Autodesk Inventor part; units mm, degrees
ref_plane "YZ Plane" through (0, 0, 0) normal (1, 0, 0) x (0, 1, 0)
ref_plane "XZ Plane" through (0, 0, 0) normal (0, 1, 0) x (-1, 0, 0)
ref_plane "XY Plane" through (0, 0, 0) normal (0, 0, 1) x (1, 0, 0)
sketch "スケッチ1" plane through (0, 0, 0) normal (0, 0, 1) x (1, 0, 0)
  point P0 (0, 0)
sketch "スケッチ2" plane through (0, 0, 0) normal (0, 0, 1) x (1, 0, 0)
  line L0 (72.5, -37.5) -> (-72.5, -37.5)
  line L1 (-72.5, -37.5) -> (-72.5, 37.5)
  line L2 (-72.5, 37.5) -> (72.5, 37.5)
  line L3 (72.5, 37.5) -> (72.5, -37.5)
  line L4 (72.5, -37.5) -> (-72.5, 37.5) construction
  line L5 (-72.5, -37.5) -> (72.5, 37.5) construction
  circle A0 centre (-48, -17) radius 6.05
  circle A1 centre (-48, -17) radius 9
  circle A2 centre (-57, -17) radius 1.6
  circle A3 centre (-48, -26) radius 1.6
  circle A4 centre (-39, -17) radius 1.6
  circle A5 centre (-48, -8) radius 1.6
  line L6 (67.5, 32.5) -> (-67.5, 32.5)
  line L7 (-67.5, 32.5) -> (-67.5, -32.5)
  line L8 (-67.5, -32.5) -> (67.5, -32.5)
  line L9 (67.5, -32.5) -> (67.5, 32.5)
  line L10 (-67.5, 32.5) -> (-67.5, 12.5) construction
  line L11 (-69.1, 32.5) -> (-69.1, 12.5)
  line L12 (-65.9, 12.5) -> (-65.9, 32.5)
  arc A6 (-65.9, 32.5) -> (-69.1, 32.5) centre (-67.5, 32.5) ccw
  arc A7 (-69.1, 12.5) -> (-65.9, 12.5) centre (-67.5, 12.5) ccw
  line L13 (-67.5, 32.5) -> (-47.5, 32.5) construction
  line L14 (-67.5, -32.5) -> (-67.5, -12.5) construction
  line L15 (-65.9, -32.5) -> (-65.9, -12.5)
  line L16 (-69.1, -12.5) -> (-69.1, -32.5)
  arc A8 (-69.1, -32.5) -> (-65.9, -32.5) centre (-67.5, -32.5) ccw
  arc A9 (-65.9, -12.5) -> (-69.1, -12.5) centre (-67.5, -12.5) ccw
  line L17 (-67.5, -32.5) -> (-47.5, -32.5) construction
  line L18 (67.5, 32.5) -> (105, 32.5) construction
  line L19 (-72.5, -17) -> (72.5, -17)
  circle A10 centre (0, -17) radius 9
  circle A11 centre (0, -17) radius 39
  line L20 (-65, 37.5) -> (65, 37.5)
  line L21 (65, 37.5) -> (65, 32.5)
  line L22 (65, 32.5) -> (-65, 32.5)
  line L23 (-65, 32.5) -> (-65, 37.5)
  line L24 (-65, 32.5) -> (0, 0)
  line L25 (0, 0) -> (65, 32.5)
  line L26 (-72.5, 0) -> (72.5, 0)
  line L27 (72.5, 0) -> (72.5, -47.5)
  line L28 (72.5, -47.5) -> (-72.5, -47.5)
  line L29 (-72.5, -47.5) -> (-72.5, 0)
  circle A12 centre (-67.5, 32.5) radius 1.6
  circle A13 centre (-67.5, -12.5) radius 1.6
  line L30 (0, 37.5) -> (0, -47.5)
  line L31 (67.5, 32.5) -> (67.5, 12.5) construction
  line L32 (69.1, 32.5) -> (69.1, 12.5)
  line L33 (65.9, 12.5) -> (65.9, 32.5)
  arc A14 (69.1, 32.5) -> (65.9, 32.5) centre (67.5, 32.5) ccw
  arc A15 (65.9, 12.5) -> (69.1, 12.5) centre (67.5, 12.5) ccw
  line L34 (67.5, -32.5) -> (67.5, -12.5) construction
  line L35 (65.9, -32.5) -> (65.9, -12.5)
  line L36 (69.1, -12.5) -> (69.1, -32.5)
  arc A16 (65.9, -32.5) -> (69.1, -32.5) centre (67.5, -32.5) ccw
  arc A17 (69.1, -12.5) -> (65.9, -12.5) centre (67.5, -12.5) ccw
  circle A18 centre (67.5, 32.5) radius 1.6
  circle A19 centre (67.5, -12.5) radius 1.6
  circle A20 centre (-57.5, -17) radius 1.6
  circle A21 centre (-57.5, 17) radius 1.6
  circle A22 centre (57.5, -17) radius 1.6
  circle A23 centre (57.5, 17) radius 1.6
  circle A24 centre (45.5961, -2) radius 6.55
  circle A25 centre (45.5961, -2) radius 9.5
  circle A26 centre (55.0961, -2) radius 1.35
  circle A27 centre (40.8461, 6.2272) radius 1.35
  circle A28 centre (40.8461, -10.2272) radius 1.35
  circle A29 centre (45.5961, -2) radius 24
  circle A30 centre (0, -17) radius 24
  line L37 (69.5961, -2) -> (21.5961, -2)
  line L38 (0, -41) -> (-72.5, -32.5)
  line L39 (0, -41) -> (72.5, -32.5)
  circle A31 centre (-37.5, -12.5) radius 1.6
  circle A32 centre (-27.5, -17) radius 1.6
  circle A33 centre (-37.5, 32.5) radius 1.6
  circle A34 centre (-27.5, 17) radius 1.6
  line L40 (-42.5, 37.5) -> (-42.5, -47.5)
  circle A35 centre (45.5961, -2) radius 12.2
  point P0 (-67.5, 22.5)
  point P1 (-67.5, -22.5)
  point P2 (-39.1422, -18.5937)
  point P3 (-39.1422, -15.4063)
  point P4 (65, 37.5)
  point P5 (67.5, 22.5)
  point P6 (67.5, -22.5)
  point P7 (-65.9, -12.5)
  point P8 (-69.1, 32.5)
  point P9 (-65, 32.5)
  point P10 (36, -2)
  point P11 (38.741, -15.0124)
  point P12 (33.8387, -0.1107)
  point P13 (63.5912, 34.2414)
  point P14 (65, 36.6)
  point P15 (-65, 36.6)
  point P16 (-63.5912, 34.2414)
  point P17 (-5.5513, -40.3492)
  point P18 (5.5513, -40.3492)
  point P19 (72.5, -32.5)
  point P20 (25.3223, 12.6611)
  point P21 (-25.3223, 12.6611)
  point P22 (-72.5, -32.5)
  point P23 (-42.5, 37.5)
  point P24 (-42.5, -36.0172)
  dimension "d15" = 18
  dimension "d56" = 19
  dimension "d60" = 48
  dimension "d0" = 145
  dimension "d1" = 75
  dimension "d5" = 12.1
  dimension "d16" = 3.2
  dimension "d19" = 360
  dimension "d21" = 5
  dimension "d22" = 20
  dimension "d23" = 90
  dimension "d24" = 3.2
  dimension "d25" = 20
  dimension "d26" = 90
  dimension "d27" = 3.2
  dimension "d36" = 20.5
  dimension "d37" = 18
  dimension "d38" = 78
  dimension "d40" = 48
  dimension "d43" = 130
  dimension "d44" = 65
  dimension "d46" = 47.5
  dimension "d47" = 3.2
  dimension "d48" = 3.2
  dimension "d49" = 10
  dimension "d50" = 10
  dimension "d51" = 17
  dimension "d52" = 17
  dimension "d55" = 13.1
  dimension "d57" = 2.7
  dimension "d58" = 360
  dimension "d59" = 48
  dimension "d62" = 15
  dimension "d65" = 30
  dimension "d70" = 30
  dimension "d71" = 24.4
extrude "押し出し1" add sketch "スケッチ2" along normal blind 10 contours L39 A16 L36 L19 L3 | L39 A30 L0 | L0 A30 L8 A11 L39 | A11 L8 A16 L39 | L19 L36 A17 A29 L26 L3 | L39 A16 L8 L9 L19 L36 | A30 L39 L30 L0 | L0 L30 L8 A30 | A11 A29 L19 L35 L8 | L8 A30 L19 A29 A11 | L26 A29 L9 A15 L32 A14 L6 L21 L2 L3 | L19 L9 A19 L36 | L30 L38 A30 L0 | L0 A30 L8 L30 | L8 L30 A10 L19 A30 | L35 L19 L9 L8 | A29 L19 A11 | A11 L19 A22 A29 | A29 L37 L9 L26 | L26 L9 A29 | L19 L35 A29 A19 L9 | A30 L38 L0 | L0 L38 A11 L8 A30 | L8 A30 L19 A10 L30 | A30 A29 L19 | L19 A10 L30 L26 A30 | L38 L40 L8 A11 | L19 A29 L35 | A11 A35 L37 L9 A17 L35 A29 L19 A22 | L19 A29 L37 A35 A11 | L21 L6 L30 L2 | L26 A35 A11 A29 L25 A23 L9 | L9 L37 A35 L26 | A29 A17 L9 L37 | A29 A23 L25 L6 L33 A15 L9 | L8 A11 A4 L19 A32 A30 | A30 L26 A29 | L8 L40 A1 A4 A11 | L35 A19 A29 | A35 L37 A11 A25 | A11 A25 A28 A26 L37 A35 | L30 L6 A33 L40 L2 | L25 A29 A11 L30 L6 | A35 L37 A26 A25 L26 | L26 A25 A27 A11 A35 | A15 L33 A18 L9 | L9 A18 L32 A15 | A30 L26 L30 A10 L19 | L19 A32 A4 A11 A31 L26 A30 | A29 L26 A35 L37 | A30 L25 A11 A29 L26 | L26 L25 A30 | A11 L19 A4 | A4 A1 A11 | A25 A11 | A11 A25 L37 A24 A26 A28 | A35 L26 A11 L37 | L30 A11 L24 L40 L6 A33 | L25 A29 | A25 A26 L37 A24 L26 | L26 A24 A25 A27 | A35 L26 A29 A11 | A11 L26 A35 | A30 L24 L26 | L26 A11 L24 A30 | L30 A30 L25 | L24 A30 L30 | A30 L30 A11 L25 | L40 A0 L19 A4 A1 | A4 L19 A1 | L19 A11 A4 | L19 A4 A1 | A1 A4 A11 | A11 L37 A25 | A11 L26 A25 L37 | L30 A30 L24 A11 | A29 A11 L25 | L26 L40 L24 A11 | A11 A31 A4 A1 L40 L26 | L40 L19 A0 | L19 A0 L40 A1 A4 | A25 L26 A24 L37 | L19 L40 A0 picked at (-42.3988, -18.41) picked at (-42.3988, -15.59)
fillet "フィレット1" radius 5 5 edges at (72.5, 37.5, 5) (72.5, -32.5, 5) (0, -41, 5) (-42.5, 37.5, 5) (-42.5, -36.0172, 5)
equation "\"d25\" = d22"
equation "\"d27\" = d24"
equation "\"d40\" = d39"
equation "\"d44\" = 0.5 * d43"
properties part number "small_plate_motor"
The listing builds one solid part. Answer for the finished solid, in the listing's coordinates (mm). Round coordinates to 2 decimals unless told otherwise and drop trailing zeros. Order: outer loops, then holes, each group sorted by start corner. A loop starts at its lowest first (then second) coordinate and runs counter-clockwise, first axis right, second up. Notation, with made-up numbers: (74.25, 31.25) -> (103.25, 31.25) arc R34 ccw to (103.25, 67.25) -> close; hole circle Ø3 at (60, -27). An arc over 180 degrees is marked (long way). Write each question's results on one line, items separated by ' | '. Start each with the question number.
Q1. Each of these flat-tipped pins is pushed along its axis until it touches: pin 1 (1.9 mm diameter, centred on x = 57.5, y = 17, fed in from -Z); pin 2 (4 mm diameter, centred on x = 45, z = 7, fed in from -Y). Where does it stop, or does it pass through?
Q2. The mould has two halves that part along X. Classify faces 1 (the flat face through (14, -1, 10)), 2 (the flat face through (-42.5, 1, 5)), 3 (the cylindrical face through (-28.68, 15.92, 4.93)): pulls with the +X half, pulls with the -X half, needs draft (parallel to the pull), parting line crosses it, or undercut.
Q3. Straight lines are drawn through the part: probe 1 along X at (y, z) = (-2, 6.5); probe 2 along X at (y, z) = (-17, 7.5); probe 3 along Y at (x, z) = (40, 7). For each, find the intervals that lie inside material, in ascending order. Write a range as from..to.
Q4. Find section B-B (y = -17). Determine the outline of the cut face in (x, z).
Q5. Find section D-D (z = 4). Give the number of separate pieces and of enclosed holes in the cut face, then the cut area to 3 significant figures.
Q6. Find section A-A (y = 17). Determine the outline of the cut face in (x, z).
Q7. Find section C-C (x = -7.5). Determine the outline of the cut face in (y, z), then the cut area to 3 significant figures.
Worked answers:
1) pin 1: passes through | pin 2: stops at y = -35.96
2) face 1: needs draft | face 2: pulls with the -X half | face 3: undercut
3) probe 1: x = -42.5..39.05, 52.15..53.75, 56.45..72.5 | probe 2: x = -42.5..-29.1, -25.9..-9, 9..55.9, 59.1..72.5 | probe 3: y = -36.31..-11.28, -9.18..-5.4, 1.4..5.18, 7.28..37.5
4) outline: (-42.5, 0) -> (-29.1, 0) -> (-29.1, 10) -> (-42.5, 10) -> close; (-25.9, 0) -> (-9, 0) -> (-9, 10) -> (-25.9, 10) -> close; (9, 0) -> (55.9, 0) -> (55.9, 10) -> (9, 10) -> close; (59.1, 0) -> (72.5, 0) -> (72.5, 10) -> (59.1, 10) -> close
5) separate pieces: 1 | enclosed holes: 13 | area: 8,120 mm2
6) outline: (-42.5, 0) -> (-29.1, 0) -> (-29.1, 10) -> (-42.5, 10) -> close; (-25.9, 0) -> (55.9, 0) -> (55.9, 10) -> (-25.9, 10) -> close; (59.1, 0) -> (72.5, 0) -> (72.5, 10) -> (59.1, 10) -> close
7) outline: (-40.12, 0) -> (-21.97, 0) -> (-21.97, 10) -> (-40.12, 10) -> close; (-12.03, 0) -> (37.5, 0) -> (37.5, 10) -> (-12.03, 10) -> close | area: 677 mm2
